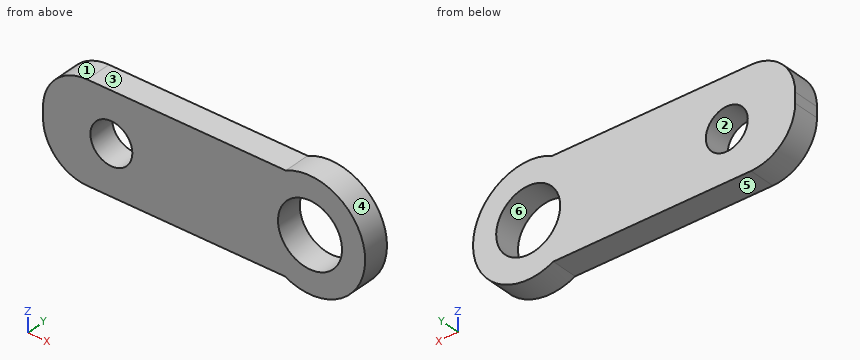
```python
from build123d import *

# Parameters (mm, degrees)
EXTRUDE_1_DEPTH     = 1.2
SKETCH_2_R          = 1.45
CUT_EXTRUDE_1_DEPTH = 13.410758407
FILLET_1_R          = 2
SKETCH_3_R          = 0.95
CUT_EXTRUDE_2_DEPTH = 13.410758407


with BuildPart() as part:
    # 草图1 → 凸台-拉伸1 (new body)
    with BuildSketch(Plane(origin=(0, 0, 0), x_dir=(1, 0, 0), z_dir=(0, 1, 0))):
        with BuildLine():
            Line((-1.096979963, -2.246471669), (-12.096979963, -2.246471669))
            Line((-12.096979963, -2.246471669), (-12.096979963, 2.224581144))
            Line((-12.096979963, 2.224581144), (-1.140718517, 2.224581144))
            ThreePointArc((-1.140718517, 2.224581144), (2.499880384, 0.024455348), (-1.096979963, -2.246471669))
        make_face()
    extrude(amount=EXTRUDE_1_DEPTH)

    # 草图2 → 切除-拉伸1 (cut, through all)
    with BuildSketch(Plane(origin=(0, 1.2, 0), x_dir=(1, 0, 0), z_dir=(0, 1, 0))):
        with Locations(Location((0, 0, 0), (0, 0, 270))):
            Circle(SKETCH_2_R)
    extrude(amount=-CUT_EXTRUDE_1_DEPTH, mode=Mode.SUBTRACT)

    # 圆角1
    fillet_1_edges = [part.edges().sort_by_distance(p)[0] for p in [
        (-12.096979963, 0.6, 2.246471669),
        (-12.096979963, 0.6, -2.224581144),
    ]]
    fillet(fillet_1_edges, radius=FILLET_1_R)

    # 草图3 → 切除-拉伸2 (cut, through all)
    with BuildSketch(Plane(origin=(0, 1.2, 0), x_dir=(1, 0, 0), z_dir=(0, 1, 0))):
        with Locations(Location((-9, -0.010945263, 0), (0, 0, 270))):
            Circle(SKETCH_3_R)
    extrude(amount=-CUT_EXTRUDE_2_DEPTH, mode=Mode.SUBTRACT)


solid = part.part
```
Geometry: final body of the model. Coordinates: model frame, mm. Face numbers are marked on the shaded views. A direction names the side the tool comes from. Coordinates: 2 decimals unless noted, no trailing zeros. Loops run counter-clockwise (first coordinate to the right, second up) from the corner with the lowest first, then second, coordinate; pieces in that order, holes last. Notation, with made-up numbers: (83, -30) -> (127, -30) arc R12 ccw to (127, -21) -> close; hole circle Ø6 at (11, 23). An arc over 180 degrees is marked (long way). Use a Markdown table: item, result. Add a question column.
(1) Mould query, pull axis X, two halves, no side actions, for the marked faces 1, 2, 3 and 4. Classes: pulls with the +X half, pulls with the -X half, needs draft (parallel to the pull), parting line crosses it, or undercut.
(2) Section query D-D, the plane x = -9. Return loops of the section in (y, z), plus the area to 3 significant figures.
(3) Access query for the marked faces 5 and 6. Directions: +Z, -Z, +X, -X, +Y, -Y. A direction counts if a zero-diameter tool reaches every point of the face in a straight line with its end or side. Return the directions, or none.
(4) Section query B-B, the plane y = 1. Return loops of the section in (x, z), plus the area to 3 significant figures.
(5) Line query: line 1 along X through (y, z) = (0.9, 0); line 2 along Z through (x, y) = (-5, 0.5); line 3 along X through (y, z) = (1.05, -0.75). Output: solid intervals per line, ascending.
(6) Pin query (flat end, axial travel): pin 1 Ø1.7 at (x, z) = (-9, 0.01) entering from -Y; pin 2 Ø0.6 at (x, y) = (-4.5, 0.5) entering from -Z; pin 3 Ø0.6 at (x, y) = (-6.5, 1) entering from +Z. Return the tip coordinate at first contact, or that it passes through.
(7) Section query A-A, the plane x = 0. Return loops of the section in (y, z).
(8) Section query C-C, the plane z = 0. Return loops of the section in (x, y).
Answer:
| question | item | result |
|---|---|---|
| 1 | face 1 | pulls with the -X half |
| 1 | face 2 | undercut |
| 1 | face 3 | needs draft |
| 1 | face 4 | parting line crosses it |
| 2 | outline | (0, -2.22) -> (1.2, -2.22) -> (1.2, -0.94) -> (0, -0.94) -> close; (0, 0.96) -> (1.2, 0.96) -> (1.2, 2.25) -> (0, 2.25) -> close |
| 2 | area | 3.09 mm^2 |
| 3 | face 5 | -Z, -X, +Y, -Y |
| 3 | face 6 | +Y, -Y |
| 4 | outline | (-12.1, -0.22) arc R2 ccw to (-10.1, -2.22) -> (-1.14, -2.22) arc R2.5 ccw (long way) to (-1.1, 2.25) -> (-10.1, 2.25) arc R2 ccw to (-12.1, 0.25) -> close; hole circle Ø1.9 at (-9, 0.01); hole circle Ø2.9 at (0, 0) |
| 4 | area | 53.1 mm^2 |
| 5 | line 1 | x = -12.1 to -9.95, -8.05 to -1.45, 1.45 to 2.5 |
| 5 | line 2 | z = -2.22 to 2.25 |
| 5 | line 3 | x = -12.03 to -9.57, -8.43 to -1.24, 1.24 to 2.38 |
| 6 | pin 1 | passes through |
| 6 | pin 2 | stops at z = -2.22 |
| 6 | pin 3 | stops at z = 2.25 |
| 7 | outline | (0, -2.5) -> (1.2, -2.5) -> (1.2, -1.45) -> (0, -1.45) -> close; (0, 1.45) -> (1.2, 1.45) -> (1.2, 2.5) -> (0, 2.5) -> close |
| 8 | outline | (-12.1, 0) -> (-9.95, 0) -> (-9.95, 1.2) -> (-12.1, 1.2) -> close; (-8.05, 0) -> (-1.45, 0) -> (-1.45, 1.2) -> (-8.05, 1.2) -> close; (1.45, 0) -> (2.5, 0) -> (2.5, 1.2) -> (1.45, 1.2) -> close |
